Build history of the part. All positions in model axes, mm. Face numbers are marked on the shaded views. A direction names the side the tool comes from. Give positions to 0.01 mm unless a question says otherwise; leave off trailing zeros. Write each loop counter-clockwise with the first axis right and the second up, starting at its lowest first coordinate (ties: lowest second). Pieces come first, ordered by that corner, then holes.
from build123d import *

# Parameters (mm, degrees)
HEX_2_DEPTH        = 6.4
THDSCHPAT_COUNT    = 8
THDSCHPAT_PITCH    = 1.766292682
SKETCH3_W          = 30.420600684
SKETCH3_H          = 33.851495499
CUT_EXTRUDE1_DEPTH = 2


with BuildPart() as part:
    # BodySke → BaseBody (revolve)
    with BuildSketch(Plane.XY):
        Polygon((0, 0), (0, 6.8985), (0.635951322, 8), (13, 8), (16, 5), (13.113248654, 0), align=None)
    revolve(axis=Axis((-12.7, 0, 0), (1, 0, 0)))

    # Sketch2 → Hex 2 (cut)
    with BuildSketch(Plane.ZY):
        Polygon((2.309401077, 4), (-2.309401077, 4), (-4.618802154, 0), (-2.309401077, -4), (2.309401077, -4), (4.618802154, 0), align=None)
    extrude(amount=-HEX_2_DEPTH, mode=Mode.SUBTRACT)

    # ThdSchSke → ThreadSchematic (revolve, cut)
    with BuildSketch(Plane.XY):
        Polygon((0.635951322, -6.8985), (-0.135327282, -8), (-0.135327282, -10), (1.407229925, -10), (1.407229925, -8), align=None)
    threadschematic = revolve(axis=Axis((-3.175, 0, 0), (1, 0, 0)), mode=Mode.SUBTRACT)

    # ThdSchPat: ThreadSchematic ×8
    with Locations(*[(i * THDSCHPAT_PITCH, 0, 0) for i in range(1, THDSCHPAT_COUNT)]):
        add(threadschematic, mode=Mode.SUBTRACT)

    # Sketch3 → Cut-Extrude1 (cut)
    with BuildSketch(Plane(origin=(0, 8, 0), x_dir=(-1, 0, 0), z_dir=(0, 1, 0))):
        with Locations((-7.768215545, -1.918808929)):
            Rectangle(SKETCH3_W, SKETCH3_H)
    extrude(amount=-CUT_EXTRUDE1_DEPTH, mode=Mode.SUBTRACT)


solid = part.part
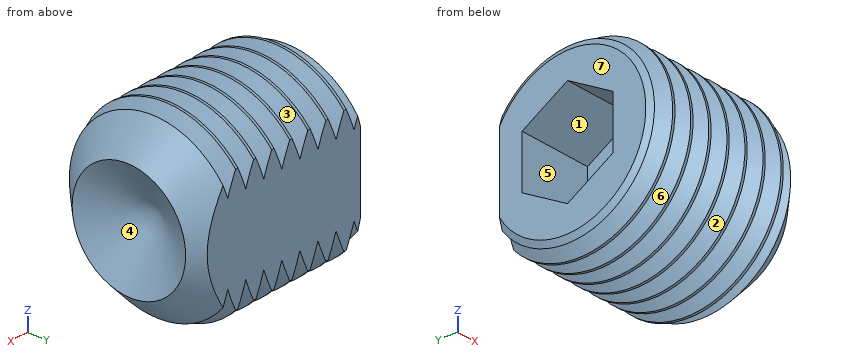
(1) Saw through at A-A, the plane x = 2. List the corners of the cut face in (y, z), plus the area to 3 significant figures.
(2) Probe line 1 (Y direction, x = 1, z = -4); line 2 (Z direction, x = 15, y = 0.5); line 3 (Z direction, x = 5, y = -2). List the from-to ranges inside material, lowest first.
(3) 3-axis set-ups, long thin cutter, end or side, ignore diameter. For the marked faces 5, 6 and 7: which of +Z, -Z, +X, -X, +Y, -Y reach the whole face in a straight line?
(4) Saw through at B-B, the plane x = 14.5. List the corners of the cut face in (y, z).
(5) Drop flat-ended pins along their axis: pin 1 (1 mm diameter, centred on x = 6, y = -6, fed in from -Z); pin 2 (3 mm diameter, centred on x = 2, y = 4.5, fed in from +Z); pin 3 (1 mm diameter, centred on y = -6.5, z = -5, fed in from +X). Give the stop position or say it passes through.
(6) Mould opens along X. For the marked faces 1, 2, 3 and 4 say: +X half, -X half, draft (parallel to the pull), parting line (faces both ways), or undercut.
Computed values:
1. outline: (6, -4.45) - (6, 4.45) arc R7.47 ccw (long way) to start; hole (-4, -2.31) - (0, -4.62) - (4, -2.31) - (4, 2.31) - (0, 4.62) - (-4, 2.31) - close
1. area: 111 mm2
2. line 1: y = -6.25 to -1.07, 1.07 to 6
2. line 2: z = -5.98 to -3.23, 3.23 to 5.98
2. line 3: z = -7.75 to -3.46, 3.46 to 7.75
3. face 5: -X
3. face 6: none
3. face 7: +Z, -Z, -X, +Y, -Y
4. outline: (6, -2.5) - (6, 2.5) arc R6.5 ccw (long way) to start; hole circle Ø4.8 at (0, 0)
5. pin 1: stops at z = -4.99
5. pin 2: stops at z = 7.4
5. pin 3: stops at x = 12.44
6. face 1: draft
6. face 2: undercut
6. face 3: undercut
6. face 4: +X half
